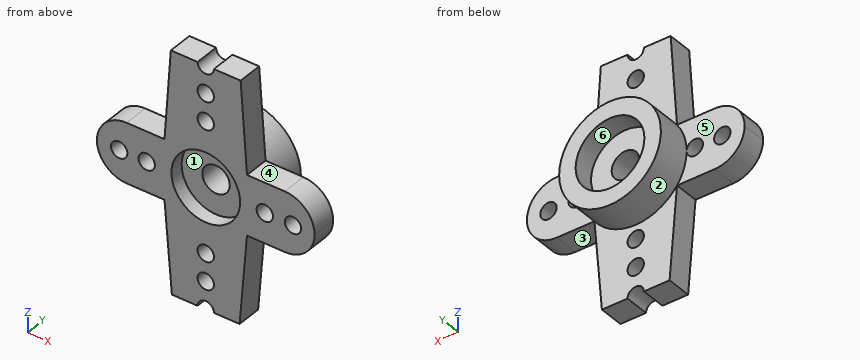
```python
from build123d import *

# Parameters (mm, degrees)
SKETCH2_R           = 2.5
SKETCH2_R_2         = 0.595
BOSS_EXTRUDE1_DEPTH = 1.8
SKETCH3_R           = 3.7
SKETCH3_R_2         = 2.5
BOSS_EXTRUDE2_DEPTH = 2.5
SKETCH4_R           = 2.5
SKETCH4_R_2         = 1
BOSS_EXTRUDE3_DEPTH = 1.8


with BuildPart() as part:
    # Sketch2 → Boss-Extrude1 (new body)
    with BuildSketch(Plane(origin=(0, 0, 0), x_dir=(1, 0, 0), z_dir=(0, 1, 0))):
        with BuildLine():
            Line((-2.460864044, 8.71), (-0.595, 8.71))
            ThreePointArc((-0.595, 8.71), (0, 8.115), (0.595, 8.71))
            Line((0.595, 8.71), (2.460864044, 8.71))
            Line((2.460864044, 8.71), (3.000462464, 2.165))
            Line((3.000462464, 2.165), (5.750462464, 2.165))
            ThreePointArc((5.750462464, 2.165), (7.281348646, 1.530886181), (7.915462464, 0))
            ThreePointArc((7.915462464, 0), (7.281348646, -1.530886181), (5.750462464, -2.165))
            Line((5.750462464, -2.165), (3.000462464, -2.165))
            Line((3.000462464, -2.165), (2.537213308, -8.71))
            Line((2.537213308, -8.71), (0.595, -8.71))
            ThreePointArc((0.595, -8.71), (0, -8.115), (-0.595, -8.71))
            Line((-0.595, -8.71), (-2.537213308, -8.71))
            Line((-2.537213308, -8.71), (-3.000462464, -2.165))
            Line((-3.000462464, -2.165), (-5.750462464, -2.165))
            ThreePointArc((-5.750462464, -2.165), (-7.281348646, -1.530886181), (-7.915462464, 0))
            ThreePointArc((-7.915462464, 0), (-7.281348646, 1.530886181), (-5.750462464, 2.165))
            Line((-5.750462464, 2.165), (-3.000462464, 2.165))
            Line((-3.000462464, 2.165), (-2.460864044, 8.71))
        make_face()
        with Locations(Location((0, 0, 0), (0, 0, 270))):
            Circle(SKETCH2_R, mode=Mode.SUBTRACT)
        with Locations(Location((-4.295, 0, 0), (0, 0, 270))):
            Circle(SKETCH2_R_2, mode=Mode.SUBTRACT)
        with Locations(Location((-6.295, 0, 0), (0, 0, 270))):
            Circle(SKETCH2_R_2, mode=Mode.SUBTRACT)
        with Locations(Location((0, 4.71, 0), (0, 0, 270))):
            Circle(SKETCH2_R_2, mode=Mode.SUBTRACT)
        with Locations(Location((0, 6.71, 0), (0, 0, 270))):
            Circle(SKETCH2_R_2, mode=Mode.SUBTRACT)
        with Locations(Location((0, -4.71, 0), (0, 0, 90))):
            Circle(SKETCH2_R_2, mode=Mode.SUBTRACT)
        with Locations(Location((0, -6.71, 0), (0, 0, 90))):
            Circle(SKETCH2_R_2, mode=Mode.SUBTRACT)
        with Locations(Location((6.345, 0, 0), (0, 0, 90))):
            Circle(SKETCH2_R_2, mode=Mode.SUBTRACT)
        with Locations(Location((4.295, 0, 0), (0, 0, 90))):
            Circle(SKETCH2_R_2, mode=Mode.SUBTRACT)
    extrude(amount=BOSS_EXTRUDE1_DEPTH)

    # Sketch3 → Boss-Extrude2 (add)
    with BuildSketch(Plane(origin=(0, 1.8, 0), x_dir=(1, 0, 0), z_dir=(0, 1, 0))):
        with Locations(Location((0, 0, 0), (0, 0, 144.187462738))):
            Circle(SKETCH3_R)
        with Locations(Location((0, 0, 0), (0, 0, 270))):
            Circle(SKETCH3_R_2, mode=Mode.SUBTRACT)
    extrude(amount=BOSS_EXTRUDE2_DEPTH)

    # Sketch4 → Boss-Extrude3 (add)
    with BuildSketch(Plane(origin=(0, 1, 0), x_dir=(-1, 0, 0), z_dir=(0, -1, 0))):
        with Locations(Location((0, 0, 0), (0, 0, 90))):
            Circle(SKETCH4_R)
        with Locations(Location((0, 0, 0), (0, 0, 90))):
            Circle(SKETCH4_R_2, mode=Mode.SUBTRACT)
    extrude(amount=-BOSS_EXTRUDE3_DEPTH)


solid = part.part
```
Read the model definition and answer for the solid it produces. Units are mm, in the model's axes. Face numbers are marked on the shaded views. A direction names the side the tool comes from. Round coordinates to 2 decimals unless told otherwise and drop trailing zeros. Write each loop counter-clockwise with the first axis right and the second up, starting at its lowest first coordinate (ties: lowest second). Pieces come first, ordered by that corner, then holes. Notation, with made-up numbers: (-27.5, 31.5) - (14.5, 31.5) arc R24 cw to (14.5, 41.5) - close; hole circle Ø4 at (45.25, 54). An arc over 180 degrees is marked (long way). One line per item, written item: value.
Q1. Straight lines are drawn through the part: line 1 (Y direction, x = 1, z = -4.5); line 2 (X direction, y = 1.1, z = -4.71) (3 decimals); line 3 (Z direction, x = -0.25, y = 3.35). For each, find the intervals that lie inside material, in ascending order. Write a range as from..to.
The answers:
line 1: y = 0..1.8
line 2: x = -2.791..-0.595, 0.595..2.791
line 3: z = -3.69..-2.49, 2.49..3.69
Q2. For a pull along Z with two mould halves and no side action, classify the marked faces 4, 5 and 6 as pulls with the +Z half, pulls with the -Z half, needs draft (parallel to the pull), parting line crosses it, or undercut.
The answers:
face 4: pulls with the +Z half
face 5: needs draft
face 6: undercut
Q3. Find section A-A (z = -4.71). Determine the outline of the cut face in (x, y) (3 decimals), and give its area (3 significant figures).
The answers:
outline: (-2.791, 0) - (-0.595, 0) - (-0.595, 1.8) - (-2.791, 1.8) - close; (0.595, 0) - (2.791, 0) - (2.791, 1.8) - (0.595, 1.8) - close
area: 7.90 mm2
Q4. Find section C-C (z = -1.25). Determine the outline of the cut face in (x, y).
The answers:
outline: (-7.52, 0) - (-2.17, 0) - (-2.17, 1) - (2.17, 1) - (2.17, 0) - (7.52, 0) - (7.52, 1.8) - (3.48, 1.8) - (3.48, 4.3) - (2.17, 4.3) - (2.17, 2.8) - (-2.17, 2.8) - (-2.17, 4.3) - (-3.48, 4.3) - (-3.48, 1.8) - (-7.52, 1.8) - close
Q5. Which of the six approach directions +Z, -Z, +X, -X, +Y, -Y give full straight-line access (tool end or side, diameter ignored) to the marked faces 1, 2 and 3?
The answers:
face 1: -Y
face 2: +Y
face 3: -Z, +X, +Y, -Y
Q6. Each of these flat-tipped pins is pushed along its axis until it touches: P1, Ø2, axis at y = 3, z = -5.5, coming from the +X side; P2, Ø0.5, axis at x = -5, y = 1.5, coming from the +Z side (3 decimals); P3, Ø3.5, axis at x = -6, z = -0.5, coming from the +Y side; P4, Ø2, axis at x = 4.5, y = 1, coming from the -Z side (3 decimals). Where does it stop, or does it pass through?
The answers:
P1: passes through
P2: stops at z = 2.165
P3: stops at y = 1.8
P4: stops at z = -2.165
Q7. Find section B-B (y = 1.3). Count the separate pieces of the cut face and the enclosed holes in it, and give its area (3 significant figures).
The answers:
separate pieces: 1
enclosed holes: 9
area: 123 mm2
